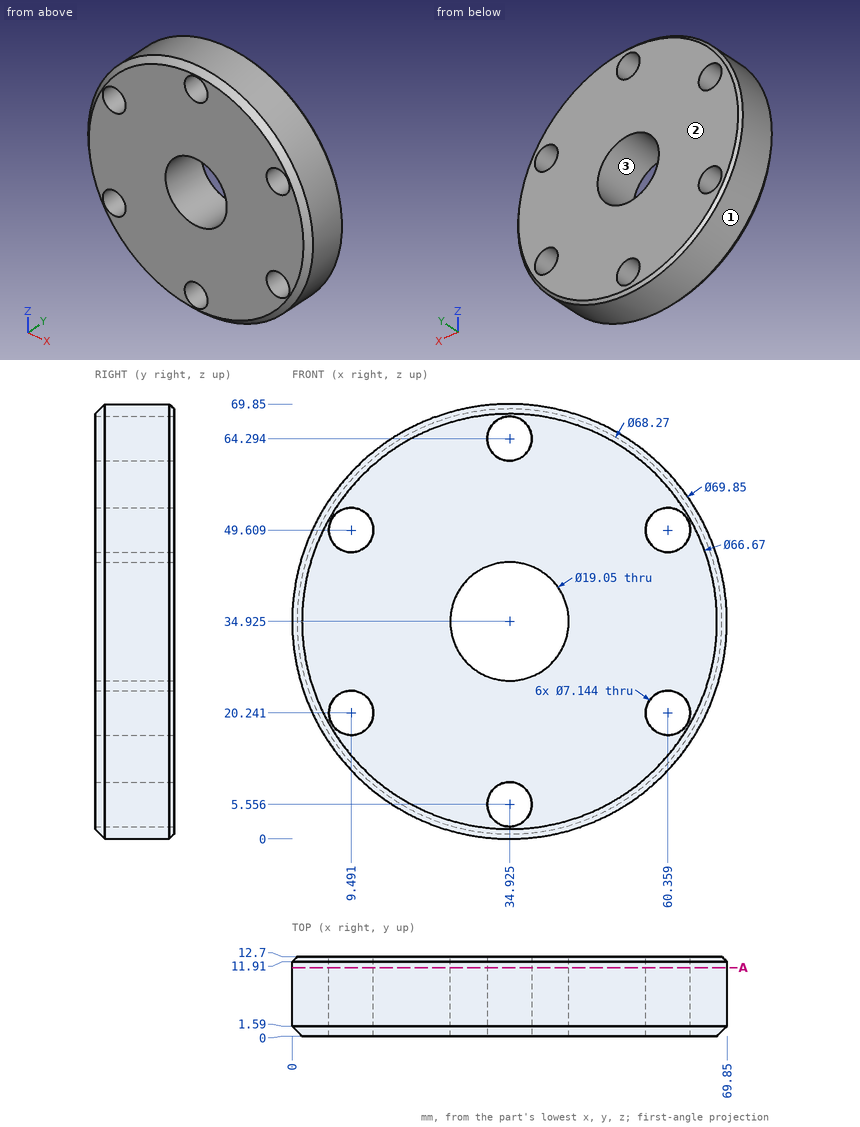
Design review of the part shown in the three views and the two pictorial views. Dimensions are in mm from the part's minimum x, y and z. Round coordinates to 2 decimals unless told otherwise and drop trailing zeros.
Q1. Add section A-A on y = 11. Give the number of separate pieces and of enclosed holes in the cut face, plus the area to 3 significant figures.
Result sheet:
separate pieces: 1
enclosed holes: 7
area: 3,310 mm2
Q2. To check wall thickness, follow line 1 along Z through (x, y) = (32.5, 9) (1 decimal); line 2 along Z through (x, y) = (38, 11) (1 decimal); line 3 along Z through (x, y) = (60.5, 11.75). State the ranges of each line that lie inside material, in increasing order.
Result sheet:
line 1: z = 0.1 to 2.9, 8.2 to 25.7, 44.1 to 61.7, 66.9 to 69.8
line 2: z = 0.1 to 3.7, 7.4 to 25.9, 43.9 to 62.5, 66.1 to 69.7
line 3: z = 11.14 to 16.67, 23.81 to 46.04, 53.18 to 58.71
Q3. Insertion check: pin 1 Ø9.5 at (x, z) = (9.49, 20.24) entering from -Y; pin 2 Ø2 at (x, y) = (10.5, 1.5) entering from -Z (1 decimal); pin 3 Ø1 at (y, z) = (9, 37) entering from +X; pin 4 Ø1 at (y, z) = (10.5, 30) entering from -X. Each pin has a flat end and moves straight along its axis. Give the tip position at first contact, or say it passes through.
Result sheet:
pin 1: stops at y = 0
pin 2: stops at z = 9
pin 3: stops at x = 69.81
pin 4: stops at x = 0.28
Q4. Mouldability with a two-part tool opening along Z and no side actions: class the marked faces 1, 2 and 3 as +Z half, -Z half, draft (parallel to the pull), parting line (faces both ways), or undercut.
Result sheet:
face 1: parting line
face 2: draft
face 3: undercut
